Verification items for the finished model (mm, model axes). Round coordinates to 2 decimals unless told otherwise and drop trailing zeros. Loops run counter-clockwise (first coordinate to the right, second up) from the corner with the lowest first, then second, coordinate; pieces in that order, holes last. Notation, with made-up numbers: M 61.25,82 L 87.25,82 A16 ccw 87.25,95 Z; hole C 40.5,-29 d8. An arc over 180 degrees is marked long. Answer as CSV lines item,"result".
Autodesk Inventor part; units mm, degrees
ref_plane "YZ Plane" through (0, 0, 0) normal (1, 0, 0) x (0, 1, 0)
ref_plane "XZ Plane" through (0, 0, 0) normal (0, 1, 0) x (-1, 0, 0)
ref_plane "XY Plane" through (0, 0, 0) normal (0, 0, 1) x (1, 0, 0)
sketch "Sketch1" plane through (0, 0, 0) normal (1, 0, 0) x (0, 1, 0)
  line L0 (75, 70) -> (-75, 70)
  line L1 (-75, 70) -> (-75, -70)
  line L2 (-75, -70) -> (75, -70)
  line L3 (75, -70) -> (75, 70)
  point P0 (0, 0)
  point P1 (75, 0)
  point P2 (0, 70)
  dimension "d0" = 140
  dimension "d1" = 150
extrude "Extrusion1" add sketch "Sketch1" along normal mid plane 5
sketch "Sketch2" plane through (2.5, 0, 0) normal (1, 0, 0) x (0, 0, -1)
  line L0 (70, 75) -> (-70, 75)
  line L1 (-10.18, 40) -> (10.18, 40)
  point P0 (0, 0)
  point P1 (0, 40)
  dimension "d4" = 20.36
  dimension "d5" = 35
hole "Hole1" at (2.5, 40, 10.18) at (2.5, 40, -10.18) direction (-1, 0, 0) diameter 2.4 depth 4
pattern_linear "Rectangular Pattern1" count 2 spacing 80 along (0, -1, 0) of "Hole1"
sketch "Sketch3" plane through (2.5, 0, 0) normal (1, 0, 0) x (0, 0, -1)
  circle A0 centre (10.18, -40) radius 1.2
  point P0 (0, 0)
  point P1 (13.0561, -20)
  point P2 (63.8461, -20)
  dimension "d16" = 50.79
  dimension "d19" = 20
  dimension "d20" = 13.0561
hole "Hole2" at (2.5, -20, -13.0561) at (2.5, -20, -63.8461) direction (-1, 0, 0) diameter 2.4 depth 4
sketch "Sketch4" plane through (2.5, 0, 0) normal (1, 0, 0) x (0, 0, -1)
  line L0 (70, 75) -> (-70, 75)
  circle A0 centre (13.0561, -20) radius 1.2
  circle A1 centre (63.8461, -20) radius 1.2
  line L1 (13.0561, -20) -> (63.8461, -20)
  point P0 (0, 0)
  point P1 (38.4511, 55)
  point P2 (38.4511, -20)
  point P3 (38.4511, 10)
  dimension "d28" = 20
  dimension "d29" = 45
hole "Hole3" at (2.5, 55, -38.4511) at (2.5, 10, -38.4511) direction (-1, 0, 0) diameter 14 depth 5
properties part number "Part_B9"
1) Go/stop test with a flat-tipped pin: pin 1 (1.2 mm diameter, centred on y = -19.5, z = -13, fed in from +X). Record where the tip stops, or that it passes through.
Here are the results:
pin 1,"stops at x = -1.5"
2) Section check C-C (z = -37.5). Record the cut outline in (x, y).
Here are the results:
outline,"M -2.5,-75 L 2.5,-75 L 2.5,3.06 L -2.5,3.06 Z; M -2.5,16.94 L 2.5,16.94 L 2.5,48.06 L -2.5,48.06 Z; M -2.5,61.94 L 2.5,61.94 L 2.5,75 L -2.5,75 Z"
3) Material ranges on probe 1 along Y at (x, z) = (2.1, -39); probe 2 along Y at (x, z) = (1.15, 10.18); probe 3 along Z at (x, y) = (-0.35, 40), recorded low to high.
Here are the results:
probe 1,"y = -75 to 3.02, 16.98 to 48.02, 61.98 to 75"
probe 2,"y = -75 to -41.2, -38.8 to 38.8, 41.2 to 75"
probe 3,"z = -70 to -11.38, -8.98 to 8.98, 11.38 to 70"
4) Section check A-A (y = 10). Record the cut outline in (x, z).
Here are the results:
outline,"M -2.5,-70 L 2.5,-70 L 2.5,-45.45 L -2.5,-45.45 Z; M -2.5,-31.45 L 2.5,-31.45 L 2.5,70 L -2.5,70 Z"
5) Draft check along Z on faces 1 (the cylindrical face through (-0.04, 48.06, -37.54)), 2 (the flat face through (0, 1, 70)), 3 (the flat face through (-2.5, -1, 1)). Enter one of: +Z half, -Z half, draft (parallel to the pull), parting line (faces both ways), or undercut.
Here are the results:
face 1,"undercut"
face 2,"+Z half"
face 3,"draft"
6) Section check B-B (x = 1.7). State how many separate pieces and enclosed holes the cut face has, plus the area to 3 significant figures.
Here are the results:
separate pieces,"1"
enclosed holes,"8"
area,"20,700 mm^2"
